Work out the finished part from the listing and answer in its coordinate system (mm). A direction names the side the tool comes from. Give positions to 0.01 mm unless a question says otherwise; leave off trailing zeros. Loops run counter-clockwise (first coordinate to the right, second up) from the corner with the lowest first, then second, coordinate; pieces in that order, holes last.
```python
from build123d import *

# Parameters (mm, degrees)
BOSS_EXTRUDE1_DEPTH = 10


with BuildPart() as part:
    # Sketch1 → Boss-Extrude1 (new body)
    with BuildSketch(Plane(origin=(0, 0, 0), x_dir=(1, 0, 0), z_dir=(0, 1, 0))):
        Polygon((0, 0), (87.513060243, 0), (79.763338482, 20), (59.763338482, 20), (59.763338482, 30), (75.888477602, 30), (48.76445144, 100), (28.76445144, 100), (28.76445144, 110), (8.76445144, 110), (8.76445144, 100), (-11.23554856, 100), (-19.274024332, 70), (-1.953516257, 70), (-1.953516257, 60), (-21.953516257, 60), (-38.030467803, 0), align=None)
    extrude(amount=BOSS_EXTRUDE1_DEPTH)


solid = part.part
```
Q1. Section A-A on x = 65.5 is taken. Give the vertices of the cut face in (y, z).
Q2. Section C-C on z = -84 is taken. Give the vertices of the cut face in (x, y), plus the area to 3 significant figures.
Q3. Given pin 1 (12 mm diameter, centred on x = 55.5, z = -95.5, fed in from +Y); pin 2 (3 mm diameter, centred on y = 5, z = -107.5, fed in from +X); pin 3 (5 mm diameter, centred on x = -2, y = 4.5, fed in from -Z); pin 4 (3 mm diameter, centred on y = 8.5, z = -37, fed in from +X), each flat-ended and moving along its own axis, determine where each tip first touches the part or whether it passes through.
Q4. Consider line 1 along Z through (x, y) = (-6, 3.25); line 2 along Z through (x, y) = (32, 7.75); line 3 along X through (y, z) = (5, -36). Determine where each line is inside the solid, lowest interval first.
Q5. Section B-B on y = 5 is taken. Give the vertices of the cut face in (x, z), plus the area to 3 significant figures.
Q6. Which of the six approach directions +Z, -Z, +X, -X, +Y, -Y give full straight-line access (tool end or side, diameter ignored) to faces 5 (the face through (28.764, 5, -105)), 6 (the face through (70, 5, -20)), 7 (the face through (8.764, 5, -105))?
Q7. Section D-D on x = 31 is taken. Give the vertices of the cut face in (y, z), plus the area to 3 significant figures.
Q8. Determine the mould class of faces 1 (the face through (68, 5, -30)), 2 (the face through (59.763, 5, -25)), 3 (the face through (24, 0, -44)), 4 (the face through (83.692, 4.93, -9.86)) for opening direction Z: +Z half, -Z half, draft (parallel to the pull), parting line (faces both ways), or undercut.
Check result:
1. outline: (0, -56.81) - (10, -56.81) - (10, -30) - (0, -30) - close; (0, -20) - (10, -20) - (10, 0) - (0, 0) - close
2. outline: (-15.52, 0) - (54.96, 0) - (54.96, 10) - (-15.52, 10) - close
2. area: 705 mm2
3. pin 1: stops at y = 10
3. pin 2: stops at x = 28.76
3. pin 3: stops at z = -100
3. pin 4: stops at x = 73.76
4. line 1: z = -100 to -70, -60 to 0
4. line 2: z = -100 to 0
4. line 3: x = -28.38 to 73.56
5. outline: (-38.03, 0) - (-21.95, -60) - (-1.95, -60) - (-1.95, -70) - (-19.27, -70) - (-11.24, -100) - (8.76, -100) - (8.76, -110) - (28.76, -110) - (28.76, -100) - (48.76, -100) - (75.89, -30) - (59.76, -30) - (59.76, -20) - (79.76, -20) - (87.51, 0) - close
5. area: 9,110 mm2
6. face 5: -Z, +X, +Y, -Y
6. face 6: +X, +Y, -Y
6. face 7: -Z, -X, +Y, -Y
7. outline: (0, -100) - (10, -100) - (10, 0) - (0, 0) - close
7. area: 1,000 mm2
8. face 1: undercut
8. face 2: undercut
8. face 3: draft
8. face 4: -Z half
